Answer from the drawing. Dimensions are ordinates in mm from the lowest x, y and z of the part. Round coordinates to 2 decimals unless told otherwise and drop trailing zeros. Loops run counter-clockwise (first coordinate to the right, second up) from the corner with the lowest first, then second, coordinate; pieces in that order, holes last. Notation, with made-up numbers: (-7.5, 77) - (34.5, 77) arc R16 ccw to (34.5, 93) - close; hole circle Ø7 at (32, -18). An arc over 180 degrees is marked (long way). One line per question, with ' | ' between items. Start each with the question number.
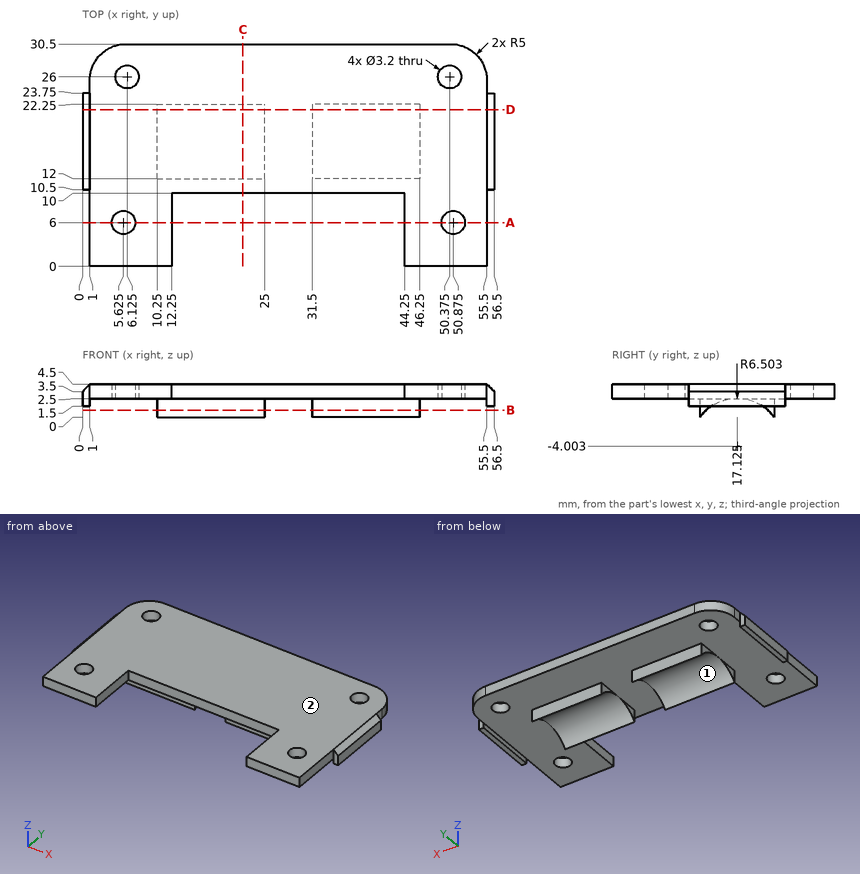
(1) Find section D-D on y = 21.5. Write down the section's boundary in (x, z).
(2) Determine the mould class of the marked faces 1 and 2 for opening direction X: pulls with the +X half, pulls with the -X half, needs draft (parallel to the pull), parting line crosses it, or undercut.
(3) Find section A-A on y = 6. Write down the section's boundary in (x, z) (3 decimals), plus the area to 3 significant figures.
(4) Consider L1, parallel to X at y = 6, z = 3.05 (3 decimals); L2, parallel to X at y = 20.5, z = 2.1; L3, parallel to X at y = 17, z = 2.05. Determine where each line is inside the solid, lowest interval first.
(5) Find section B-B on z = 0.95. Write down the section's boundary in (x, y).
(6) Each of these flat-tipped pins is pushed along its axis until it touches: P1, Ø4, axis at x = 50.375, y = 26, coming from the +Z side; P2, Ø1.6, axis at y = 7, z = 3.5, coming from the -X side; P3, Ø6, axis at x = 23, y = 17, coming from the -Z side. Where does it stop, or does it pass through?
(7) Find section C-C on x = 22. Write down the section's boundary in (y, z) (3 decimals).
Answer below:
1) outline: (0, 1.5) - (1, 1.5) - (1, 2.5) - (10.25, 2.5) - (10.25, 0.81) - (25, 0.81) - (25, 2.5) - (31.5, 2.5) - (31.5, 0.81) - (46.25, 0.81) - (46.25, 2.5) - (55.5, 2.5) - (55.5, 1.5) - (56.5, 1.5) - (56.5, 3.5) - (55.5, 4.5) - (1, 4.5) - (0, 3.5) - close
2) face 1: undercut | face 2: needs draft
3) outline: (1, 2.5) - (4.025, 2.5) - (4.025, 4.5) - (1, 4.5) - close; (7.225, 2.5) - (12.25, 2.5) - (12.25, 4.5) - (7.225, 4.5) - close; (44.25, 2.5) - (49.275, 2.5) - (49.275, 4.5) - (44.25, 4.5) - close; (52.475, 2.5) - (55.5, 2.5) - (55.5, 4.5) - (52.475, 4.5) - close | area: 32.2 mm2
4) L1: 1 to 4.025, 7.225 to 12.25, 44.25 to 49.275, 52.475 to 55.5 | L2: 0 to 1, 10.25 to 25, 31.5 to 46.25, 55.5 to 56.5 | L3: 0 to 1, 55.5 to 56.5
5) outline: (10.25, 12) - (25, 12) - (25, 12.91) - (10.25, 12.91) - close; (10.25, 21.34) - (25, 21.34) - (25, 22.25) - (10.25, 22.25) - close; (31.5, 12) - (46.25, 12) - (46.25, 12.91) - (31.5, 12.91) - close; (31.5, 21.34) - (46.25, 21.34) - (46.25, 22.25) - (31.5, 22.25) - close
6) P1: z = 4.5 | P2: x = 1 | P3: z = 1.7
7) outline: (10, 2.5) - (12, 2.5) - (12, 0) arc R6.503 cw to (22.25, 0) - (22.25, 2.5) - (30.5, 2.5) - (30.5, 4.5) - (10, 4.5) - close
